from build123d import *

# Parameters (mm, degrees)
SCHIZZO1_R                   = 5
SCHIZZO1_R_2                 = 7.5
ESTRUSIONE_ESTRUSIONE1_DEPTH = 3
SCHIZZO3_W                   = 10
SCHIZZO3_H                   = 6
ESTRUSIONE_ESTRUSIONE2_DEPTH = 10
SCHIZZO4_R                   = 2.534735547
TAGLIO_ESTRUSIONE1_DEPTH     = 9
RACCORDO1_R                  = 5
RACCORDO1_OF_SPECCHIA1_R     = 5


with BuildPart() as part:
    # Schizzo1 → Estrusione-Estrusione1 (new body)
    with BuildSketch(Plane(origin=(0, 0, 0), x_dir=(1, 0, 0), z_dir=(0, 1, 0))):
        with BuildLine():
            Line((-56.568542495, 20), (56.568542495, 20))
            ThreePointArc((56.568542495, 20), (60, 0), (56.568542495, -20))
            Line((56.568542495, -20), (-56.568542495, -20))
            ThreePointArc((-56.568542495, -20), (-60, 0), (-56.568542495, 20))
        make_face()
        with Locations(Location((45, 0, 0), (0, 0, 270))):
            Circle(SCHIZZO1_R, mode=Mode.SUBTRACT)
        with Locations(Location((-45, 0, 0), (0, 0, 270))):
            Circle(SCHIZZO1_R, mode=Mode.SUBTRACT)
        with Locations(Location((0, 0, 0), (0, 0, 270))):
            Circle(SCHIZZO1_R_2, mode=Mode.SUBTRACT)
    extrude(amount=ESTRUSIONE_ESTRUSIONE1_DEPTH)

    # Schizzo3 → Estrusione-Estrusione2 (add)
    with BuildSketch(Plane(origin=(0, 3, 0), x_dir=(1, 0, 0), z_dir=(0, 1, 0))):
        with Locations((-25, 0)):
            Rectangle(SCHIZZO3_W, SCHIZZO3_H)
    estrusione_estrusione2 = extrude(amount=ESTRUSIONE_ESTRUSIONE2_DEPTH)

    # Schizzo4 → Taglio-Estrusione1 (cut)
    with BuildSketch(Plane.XY.offset(3)):
        with Locations((-25, 8)):
            Circle(SCHIZZO4_R)
    taglio_estrusione1 = extrude(amount=-TAGLIO_ESTRUSIONE1_DEPTH, mode=Mode.SUBTRACT)

    # Raccordo1
    raccordo1_edges = [part.edges().sort_by_distance(p)[0] for p in [
        (-20, 13, 0),
        (-30, 13, 0),
    ]]
    fillet(raccordo1_edges, radius=RACCORDO1_R - 0.0001)  # a hair under: the kernel refuses the full size

    # Specchia1: Estrusione-Estrusione2, Taglio-Estrusione1 across plane
    add(estrusione_estrusione2.mirror(Plane(origin=(0, 0, 0), x_dir=(0, 0, 1), z_dir=(1, 0, 0))))
    add(taglio_estrusione1.mirror(Plane(origin=(0, 0, 0), x_dir=(0, 0, 1), z_dir=(1, 0, 0))), mode=Mode.SUBTRACT)

    # Raccordo1 of Specchia1
    raccordo1_of_specchia1_edges = [part.edges().sort_by_distance(p)[0] for p in [
        (20, 13, 0),
        (30, 13, 0),
    ]]
    fillet(raccordo1_of_specchia1_edges, radius=RACCORDO1_OF_SPECCHIA1_R - 0.0001)  # a hair under: the kernel refuses the full size


solid = part.part
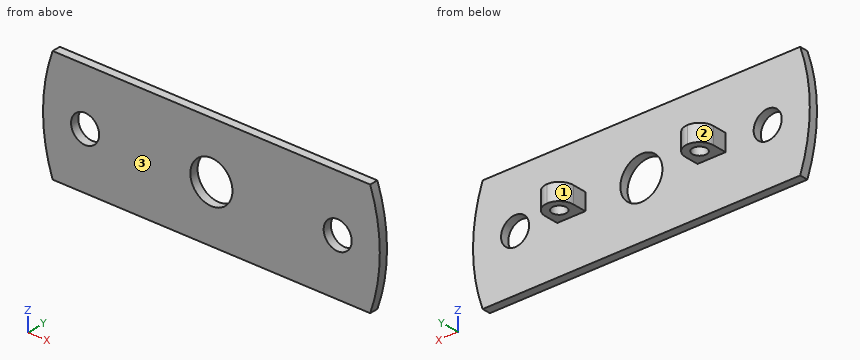
Could you check a few things on this model? Use its own coordinates, in mm. Face numbers are marked on the shaded views. Round coordinates to 2 decimals unless told otherwise and drop trailing zeros. Order: outer loops, then holes, each group sorted by start corner. A loop starts at its lowest first (then second) coordinate and runs counter-clockwise, first axis right, second up.
Q1. Imagine slicing it at A-A, the plane z = 0. State how many separate pieces and enclosed holes the cut face has, then the cut area to 3 significant figures.
Geometry says:
separate pieces: 4
enclosed holes: 2
area: 393 mm2
Q2. Imagine slicing it at B-B, the plane x = -45. List the corners of the cut face in (y, z) for me, then the cut area to 3 significant figures.
Geometry says:
outline: (0, -20) - (3, -20) - (3, -5) - (0, -5) - close; (0, 5) - (3, 5) - (3, 20) - (0, 20) - close
area: 90.0 mm2
Q3. Please list where these lines run through material, in increasing order: probe 1 along X at (y, z) = (2.1, 0); probe 2 along Y at (x, z) = (25, 0.4); probe 3 along X at (y, z) = (9.25, 1.5).
Geometry says:
probe 1: x = -60 to -50, -40 to -7.5, 7.5 to 40, 50 to 60
probe 2: y = 0 to 5.47, 10.53 to 13
probe 3: x = -29.84 to -27.21, -22.79 to -20.16, 20.16 to 22.79, 27.21 to 29.84
Q4. Imagine slicing it at C-C, the plane y = 11.75. List the corners of the cut face in (x, z) for me, then the cut area to 3 significant figures.
Geometry says:
outline: (-28.31, -3) - (-21.69, -3) - (-21.69, 3) - (-28.31, 3) - close; (21.69, -3) - (28.31, -3) - (28.31, 3) - (21.69, 3) - close
area: 79.4 mm2
Q5. I'm going to push flat-ended pins straight in: P1, Ø3, axis at x = -24, y = 8, coming from the -Z side; P2, Ø6, axis at x = 25, y = 8, coming from the +Z side; P3, Ø4, axis at y = 4.5, z = 1, coming from the -X side; P4, Ø4, axis at y = 6, z = 0, coming from the +X side. Where does each tip first touch, or does it pass through?
Geometry says:
P1: passes through
P2: stops at z = 3
P3: stops at x = -60
P4: stops at x = 30
Q6. Imagine slicing it at D-D, the plane x = 35.5. List the corners of the cut face in (y, z) for me.
Geometry says:
outline: (0, -20) - (3, -20) - (3, 20) - (0, 20) - close
Q7. Thinking about a two-plate mould opening in X: for the marked faces 1, 2 and 3, which applies, released by +X, released by -X, zero draft, split by the parting line, or undercut?
Geometry says:
face 1: undercut
face 2: released by -X
face 3: zero draft
